The listing builds one solid part. Answer for the finished solid, in the listing's coordinates (mm). Face numbers are marked on the shaded views. Give positions to 0.01 mm unless a question says otherwise; leave off trailing zeros. Write each loop counter-clockwise with the first axis right and the second up, starting at its lowest first coordinate (ties: lowest second). Pieces come first, ordered by that corner, then holes.
Autodesk Inventor part; units mm, degrees
ref_plane "YZ Plane" through (0, 0, 0) normal (1, 0, 0) x (0, 1, 0)
ref_plane "XZ Plane" through (0, 0, 0) normal (0, 1, 0) x (-1, 0, 0)
ref_plane "XY Plane" through (0, 0, 0) normal (0, 0, 1) x (1, 0, 0)
sketch "Sketch1" plane through (0, 0, 0) normal (0, 0, 1) x (1, 0, 0)
  line L0 (-41, -2.5) -> (41, -2.5)
  line L1 (41, -2.5) -> (41, 2.5)
  line L2 (41, 2.5) -> (-41, 2.5)
  line L3 (-41, 2.5) -> (-41, -2.5)
  line L4 (-41, -2.5) -> (41, 2.5) construction
  line L5 (41, -2.5) -> (-41, 2.5) construction
  point P0 (0, 0)
  dimension "d0" = 82
  dimension "d1" = 5
extrude "Extrusion1" add sketch "Sketch1" along normal blind 25
chamfer "Chamfer1" distance 1.5 angle 45 1 edges at (0, -2.5, 0)
fillet "Fillet1" radius 5 2 edges at (-41, 0, 25) (41, 0, 25)
sketch "Sketch2" plane through (-41, 2.5, 0) normal (0, 1, 0) x (1, 0, 0)
  circle A0 centre (10, -17) radius 3 construction
  circle A1 centre (72, -17) radius 3 construction
  line L0 (77, -25) -> (5, -25) construction
  line L1 (0, 0) -> (0, -20) construction
  line L2 (82, 0) -> (82, -20) construction
  point P0 (41, 0)
  dimension "d8" = 6
  dimension "d9" = 6
  dimension "d10" = 8
  dimension "d11" = 10
  dimension "d12" = 10
  dimension "d13" = 8
hole "Hole1" at (-31, 2.5, 17) at (31, 2.5, 17) direction (0, -1, 0) diameter 5 end through all
thread "Thread1"
thread "Thread2"
fillet "Fillet2" radius 1 5 edges at (-39.5355, -2.5, 23.5355) (0, -2.5, 25) (39.5355, -2.5, 23.5355) (41, -2.5, 10.75) (-41, -2.5, 10.75)
properties part number "BearingHousing_Jack" material "Steel, Galvanized"
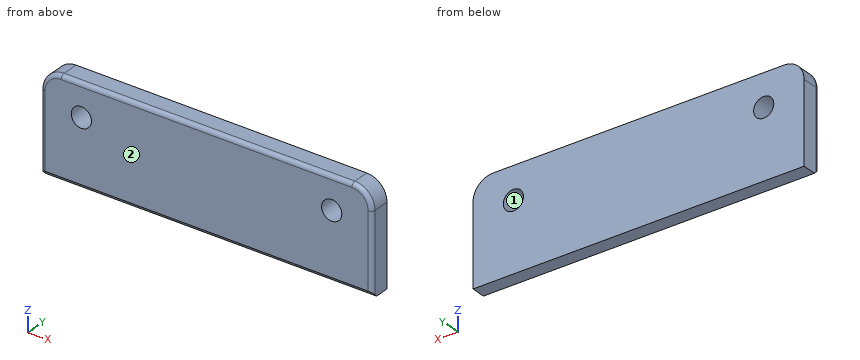
Item 1: A cutting plane is placed at A-A, the plane x = -31. Give the vertices of the cut face in (y, z), plus the area to 3 significant figures.
Conclusion:
outline: (-2.5, 1.5) - (-1, 0) - (2.5, 0) - (2.5, 14.5) - (-2.5, 14.5) - close; (-2.5, 19.5) - (2.5, 19.5) - (2.5, 25) - (-1.5, 25) arc R1 ccw to (-2.5, 24) - close
area: 98.7 mm2
Item 2: Consider probe 1 along X at (y, z) = (-1.25, 17); probe 2 along Z at (x, y) = (-31, 0); probe 3 along X at (y, z) = (-0.45, 18). Determine where each line is inside the solid, lowest interval first.
Conclusion:
probe 1: x = -41 to -33.5, -28.5 to 28.5, 33.5 to 41
probe 2: z = 0 to 14.5, 19.5 to 25
probe 3: x = -41 to -33.29, -28.71 to 28.71, 33.29 to 41
Item 3: Determine the mould class of the marked faces 1 and 2 for opening direction X: pulls with the +X half, pulls with the -X half, needs draft (parallel to the pull), parting line crosses it, or undercut.
Conclusion:
face 1: undercut
face 2: needs draft
Item 4: A cutting plane is placed at B-B, the plane z = 17. Give the vertices of the cut face in (x, y), plus the area to 3 significant figures.
Conclusion:
outline: (-41, -1.5) arc R1 ccw to (-40, -2.5) - (-33.5, -2.5) - (-33.5, 2.5) - (-41, 2.5) - close; (-28.5, -2.5) - (28.5, -2.5) - (28.5, 2.5) - (-28.5, 2.5) - close; (33.5, -2.5) - (40, -2.5) arc R1 ccw to (41, -1.5) - (41, 2.5) - (33.5, 2.5) - close
area: 360 mm2
